Autodesk Inventor part; units mm, degrees
ref_plane "YZ Plane" through (0, 0, 0) normal (1, 0, 0) x (0, 1, 0)
ref_plane "XZ Plane" through (0, 0, 0) normal (0, 1, 0) x (-1, 0, 0)
ref_plane "XY Plane" through (0, 0, 0) normal (0, 0, 1) x (1, 0, 0)
sketch "Sketch1" plane through (0, 0, 0) normal (0, 1, 0) x (-1, 0, 0)
  line L0 (0, 0) -> (6.35, 0)
  line L1 (6.35, 0) -> (6.35, -88.9)
  line L2 (6.35, -88.9) -> (0, -88.9)
  line L3 (0, -88.9) -> (0, 0)
  dimension "d0" = 6.35
  dimension "d1" = 88.9
extrude "Extrusion1" add sketch "Sketch1" along normal blind 3.175
sketch "Sketch2" plane through (0, 3.175, 0) normal (0, 1, 0) x (1, 0, 0)
  circle A0 centre (-3.175, -2.4668) radius 3.9335
  circle A1 centre (-3.175, 91.0782) radius 3.937
  point P0 (0, 0)
  dimension "d4" = 7.8671
  dimension "d5" = 7.874
extrude "Extrusion2" add sketch "Sketch2" against normal blind 3.175
sketch "Sketch3" plane through (0, 3.175, 0) normal (0, 1, 0) x (1, 0, 0)
  circle A0 centre (-3.277, 91.3462) radius 1.6256
  circle A1 centre (-3.277, -2.6864) radius 1.6256
  point P0 (0, 0)
  dimension "d8" = 3.2512
  dimension "d9" = 3.2512
extrude "Extrusion3" cut sketch "Sketch3" against normal blind 3.175
properties part number "linkage arm"
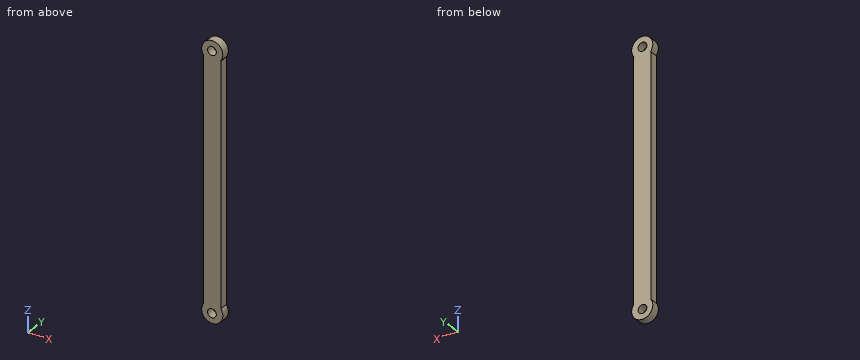
Geometry: final body of the model. Coordinates: model frame, mm. Coordinates: 2 decimals unless noted, no trailing zeros. Order: outer loops, then holes, each group sorted by start corner. A loop starts at its lowest first (then second) coordinate and runs counter-clockwise, first axis right, second up.
(1) Section query C-C (z = -72). Return the cut outline in (x, y) (3 decimals).
(2) First-contact query: pin 1 (1.5 mm diameter, centred on x = -6, y = 0.5, fed in from -Z). Flat tip, straight axial feed; report the tip coordinate or a pass-through.
(3) Section query B-B (x = -3). Return the cut outline in (y, z) (3 decimals), plus the area to 3 significant figures.
(4) Material intervals for probe 1 along Z at (x, y) = (-2.75, 2.45); probe 2 along Z at (x, y) = (-3.25, 1.8); probe 3 along X at (y, z) = (1.7, -83), sorted ascending.
(5) Section query A-A (y = 2). State how many separate pieces and enclosed holes the cut face has, plus the area to 3 significant figures.
Solution:
1. outline: (-6.35, 0) - (0, 0) - (0, 3.175) - (-6.35, 3.175) - close
2. pin 1: stops at z = -94.42
3. outline: (0, -95.011) - (3.175, -95.011) - (3.175, -92.948) - (0, -92.948) - close; (0, -89.744) - (3.175, -89.744) - (3.175, 1.085) - (0, 1.085) - close; (0, 4.288) - (3.175, 4.288) - (3.175, 6.396) - (0, 6.396) - close
3. area: 302 mm2
4. probe 1: z = -94.99 to -92.88, -89.81 to 1.15, 4.22 to 6.38
4. probe 2: z = -95.01 to -92.97, -89.72 to 1.06, 4.31 to 6.4
4. probe 3: x = -6.35 to 0
5. separate pieces: 1
5. enclosed holes: 2
5. area: 631 mm2
